For this review, take the finished solid that the model builds, in its own axes (mm). A direction names the side the tool comes from. Coordinates: 2 decimals unless noted, no trailing zeros. Order: outer loops, then holes, each group sorted by start corner. A loop starts at its lowest first (then second) coordinate and runs counter-clockwise, first axis right, second up. Notation, with made-up numbers: (-10, 11.25) -> (-6, 11.25) arc R32 cw to (-6, 39.25) -> close; hole circle Ø3 at (61.5, 11). An arc over 180 degrees is marked (long way). Return JSON: item names as keys, results as strings. Group by question number.
Item 1: For line 1 along X through (y, z) = (6.25, 31) (3 decimals); line 2 along X through (y, z) = (7.75, 56.5) (3 decimals); line 3 along Z through (x, y) = (42.5, 7), list the stretches that pass through material, from the lowest coordinate up.
Item 2: Insertion check: pin 1 (3 mm diameter, centred on y = 1.5, z = 53.5, fed in from +X) (3 decimals); pin 2 (3 mm diameter, centred on x = 71, z = 26.5, fed in from -Y). Each pin has a flat end and moves straight along its axis. Give the tip position at first contact, or say it passes through.
Item 3: Machinability: for faces 5 (the cylindrical face through (73.645, 3.131, 23.878)), 6 (the flat face through (84.626, 1.077, 72.077)), which of the approach directions +Z, -Z, +X, -X, +Y, -Y give a long, thin tool a straight path to every point of the face, cutting with its end or side? Answer none if there is none.
Item 4: Take a section at B-B (z = 26.5). Write out the cut boundary in (x, y) (3 decimals), then the cut area to 3 significant figures.
Item 5: Take a section at A-A (z = 69). Write out the cut boundary in (x, y) (3 decimals).
Item 6: Draft analysis for pull direction Y (two halves, no side actions). For faces 1 (the flat face through (58, 12.7, 47)), 2 (the flat face through (57.528, 0.776, 72.252)), 3 (the flat face through (28.575, 6, 48)), 4 (the conical face through (41.718, 6.331, 52.733)), state which applies: +Y half, -Y half, draft (parallel to the pull), parting line (faces both ways), or undercut.
Item 7: Take a section at D-D (y = 5). Count the separate pieces of the cut face and the enclosed holes in it, then the cut area to 3 significant figures.
Item 8: Take a section at C-C (y = 10.25). Write out the cut boundary in (x, z) (3 decimals), then the cut area to 3 significant figures.
```python
from build123d import *

# Parameters (mm, degrees)
F0_W           = 57.15
F0_H           = 50.8
F1_DEPTH       = 12.7
F2_D           = 6.7564
F2_CBORE_D     = 9.525
F2_CBORE_DEPTH = 6.35
F4_D           = 5.1054
F4_DEPTH       = 19.05
F4_TIP         = 1.5338169022
F5_SIZE        = 1.5748
F6_ANGLE       = 180


with BuildPart() as f1:
    # F0 (on Front) → F1 (new body)
    with BuildSketch(Plane.XZ):
        Rectangle(F0_W, F0_H)
    extrude(amount=-F1_DEPTH)

    # F2 (through all)
    with Locations(Plane.XZ):
        with Locations((-15.875, 19.05), (15.875, 19.05)):
            CounterBoreHole(F2_D / 2, F2_CBORE_D / 2, F2_CBORE_DEPTH)

    # F4
    with Locations(Plane(origin=(0, 0, -25.4), x_dir=(1, 0, 0), z_dir=(0, 0, -1))):
        with Locations((15.875, -6.35), (-15.875, -6.35)):
            Hole(F4_D / 2, depth=F4_DEPTH)
            with Locations((0, 0, -(F4_DEPTH + F4_TIP / 2))):  # 118° drill point
                Cone(0, F4_D / 2, F4_TIP, mode=Mode.SUBTRACT)

    # F5
    f5_edges = [f1.edges().sort_by_distance(p)[0] for p in [
        (28.575, 12.7, 0),
        (28.575, 0, 0),
        (-28.575, 0, 0),
        (-28.575, 12.7, 0),
        (0, 0, -25.4),
        (-28.575, 6.35, -25.4),
        (0, 12.7, -25.4),
        (28.575, 6.35, -25.4),
        (28.575, 6.35, 25.4),
        (-28.575, 6.35, 25.4),
        (0, 0, 25.4),
        (0, 12.7, 25.4),
    ]]
    chamfer(f5_edges, length=F5_SIZE)


with BuildPart() as f1_1:
    # F6: moved
    add(f1.part.rotate(Axis((28.575, 6.35, 23.8252), (0, 1, 0)), F6_ANGLE))


solid = f1_1.part
```
Findings below:
{
 "1": {"line 1": "x = 28.575 to 37.161, 45.389 to 68.911, 77.139 to 85.725", "line 2": "x = 28.575 to 39.14, 43.41 to 70.89, 75.16 to 85.725", "line 3": "z = 22.25 to 25.45, 31.75 to 53.3"},
 "2": {"pin 1": "stops at x = 85.725", "pin 2": "stops at y = 6.35"},
 "3": {"face 5": "-Y", "face 6": "+Z, +X, -Y"},
 "4": {"outline": "(28.575, 1.575) -> (30.15, 0) -> (37.001, 0) -> (37.001, 6.35) -> (38.629, 6.35) -> (38.629, 12.7) -> (30.15, 12.7) -> (28.575, 11.125) -> close; (43.921, 6.35) -> (45.549, 6.35) -> (45.549, 0) -> (68.751, 0) -> (68.751, 6.35) -> (70.379, 6.35) -> (70.379, 12.7) -> (43.921, 12.7) -> close; (75.671, 6.35) -> (77.299, 6.35) -> (77.299, 0) -> (84.15, 0) -> (85.725, 1.575) -> (85.725, 11.125) -> (84.15, 12.7) -> (75.671, 12.7) -> close", "area": "545 mm2"},
 "5": {"outline": "(28.575, 1.575) -> (30.15, 0) -> (84.15, 0) -> (85.725, 1.575) -> (85.725, 11.125) -> (84.15, 12.7) -> (30.15, 12.7) -> (28.575, 11.125) -> close; hole circle Ø5.105 at (41.275, 6.35); hole circle Ø5.105 at (73.025, 6.35)"},
 "6": {"face 1": "+Y half", "face 2": "-Y half", "face 3": "draft", "face 4": "undercut"},
 "7": {"separate pieces": "1", "enclosed holes": "2", "area": "2,590 mm2"},
 "8": {"outline": "(28.575, 23.825) -> (30.15, 22.25) -> (84.15, 22.25) -> (85.725, 23.825) -> (85.725, 71.476) -> (84.15, 73.05) -> (30.15, 73.05) -> (28.575, 71.476) -> close; hole circle Ø6.756 at (41.275, 28.6); hole circle Ø6.756 at (73.025, 28.6)", "area": "2,830 mm2"}
}
